Geometry: final body of the model. Coordinates: model frame, mm. Give positions to 0.01 mm unless a question says otherwise; leave off trailing zeros. Order: outer loops, then holes, each group sorted by start corner. A loop starts at its lowest first (then second) coordinate and runs counter-clockwise, first axis right, second up. Notation, with made-up numbers: (61, 65) - (106, 65) arc R15 ccw to (106, 77) - close; hole circle Ø1 at (39.25, -4). An arc over 180 degrees is marked (long way). One line per question, with ' | ' between items. Start each with the question number.
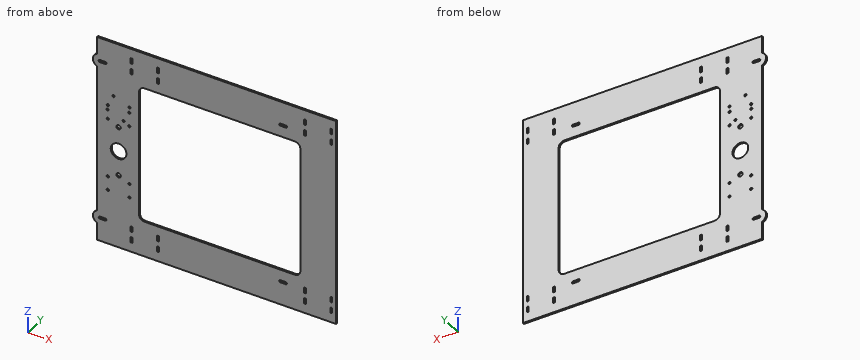
from build123d import *

# Parameters (mm, degrees)
SKETCH1_W           = 434.18
SKETCH1_H           = 380
BOSS_EXTRUDE1_DEPTH = 3
SKETCH2_W           = 250
SKETCH2_H           = 250
CUT_EXTRUDE1_DEPTH  = 4
SKETCH3_W           = 3
SKETCH3_H           = 10
CUT_EXTRUDE2_DEPTH  = 4
SKETCH6_R           = 14.2875
SKETCH6_R_2         = 2
SKETCH6_R_3         = 2.083333333
SKETCH6_R_4         = 4
CUT_EXTRUDE3_DEPTH  = 4
SKETCH7_W           = 83.283399819
SKETCH7_H           = 250
CUT_EXTRUDE4_DEPTH  = 4
FILLET1_R           = 10
CUT_EXTRUDE5_DEPTH  = 4
SKETCH9_R           = 12.5
BOSS_EXTRUDE2_DEPTH = 3


with BuildPart() as part:
    # Sketch1 → Boss-Extrude1 (new body)
    with BuildSketch(Plane(origin=(0, 0, 0), x_dir=(1, 0, 0), z_dir=(0, 1, 0))):
        Rectangle(SKETCH1_W, SKETCH1_H)
    extrude(amount=BOSS_EXTRUDE1_DEPTH)

    # Sketch2 → Cut-Extrude1 (cut, through all)
    with BuildSketch(Plane(origin=(0, 3, 0), x_dir=(1, 0, 0), z_dir=(0, 1, 0))):
        with Locations((27.09, 0)):
            Rectangle(SKETCH2_W, SKETCH2_H)
    extrude(amount=-CUT_EXTRUDE1_DEPTH, mode=Mode.SUBTRACT)

    # Sketch3 → Cut-Extrude2 (cut, through all)
    with BuildSketch(Plane(origin=(0, 3, 0), x_dir=(1, 0, 0), z_dir=(0, 1, 0))):
        with Locations((160.59, -147.5)):
            Rectangle(SKETCH3_W, SKETCH3_H)
        with Locations((160.59, -167.5)):
            Rectangle(SKETCH3_W, SKETCH3_H)
        with Locations((208.59, -147.5)):
            Rectangle(SKETCH3_W, SKETCH3_H)
        with Locations((208.59, -167.5)):
            Rectangle(SKETCH3_W, SKETCH3_H)
        with Locations((-154.41, -147.5)):
            Rectangle(SKETCH3_W, SKETCH3_H)
        with Locations((-154.41, -167.5)):
            Rectangle(SKETCH3_W, SKETCH3_H)
        with Locations((-106.41, -167.5)):
            Rectangle(SKETCH3_W, SKETCH3_H)
        with Locations((-106.41, -147.5)):
            Rectangle(SKETCH3_W, SKETCH3_H)
        with Locations((208.59, 147.5)):
            Rectangle(SKETCH3_W, SKETCH3_H)
        with Locations((208.59, 167.5)):
            Rectangle(SKETCH3_W, SKETCH3_H)
        with Locations((160.59, 167.5)):
            Rectangle(SKETCH3_W, SKETCH3_H)
        with Locations((160.59, 147.5)):
            Rectangle(SKETCH3_W, SKETCH3_H)
        with Locations((-106.41, 147.5)):
            Rectangle(SKETCH3_W, SKETCH3_H)
        with Locations((-106.41, 167.5)):
            Rectangle(SKETCH3_W, SKETCH3_H)
        with Locations((-154.41, 167.5)):
            Rectangle(SKETCH3_W, SKETCH3_H)
        with Locations((-154.41, 147.5)):
            Rectangle(SKETCH3_W, SKETCH3_H)
    extrude(amount=-CUT_EXTRUDE2_DEPTH, mode=Mode.SUBTRACT)

    # Sketch6 → Cut-Extrude3 (cut, through all)
    with BuildSketch(Plane(origin=(0, 3, 0), x_dir=(1, 0, 0), z_dir=(0, 1, 0))):
        with Locations((-177.91, 10)):
            Circle(SKETCH6_R)
        with Locations((-197.793356941, -60.788209542)):
            Circle(SKETCH6_R_2)
        with Locations((-187.137790458, -89.899356941)):
            Circle(SKETCH6_R_2)
        with Locations((-158.026643059, -79.243790458)):
            Circle(SKETCH6_R_2)
        with Locations((-168.682209542, -50.132643059)):
            Circle(SKETCH6_R_2)
        with Locations((-158.345, 64.0505)):
            Circle(SKETCH6_R_3)
        with Locations((-197.475, 64.0505)):
            Circle(SKETCH6_R_3)
        with Locations((-197.475, -44.0505)):
            Circle(SKETCH6_R_3)
        with Locations((-158.345, -44.0505)):
            Circle(SKETCH6_R_3)
        with Locations((-197.475, 89.4505)):
            Circle(SKETCH6_R_3)
        with Locations((-158.345, 89.4505)):
            Circle(SKETCH6_R_3)
        with Locations((-158.345, -69.4505)):
            Circle(SKETCH6_R_3)
        with Locations((-197.475, -69.4505)):
            Circle(SKETCH6_R_3)
        with Locations((-177.91, -35)):
            Circle(SKETCH6_R_4)
        with Locations((-177.91, 55)):
            Circle(SKETCH6_R_4)
    extrude(amount=-CUT_EXTRUDE3_DEPTH, mode=Mode.SUBTRACT)

    # Sketch7 → Cut-Extrude4 (cut, through all)
    with BuildSketch(Plane(origin=(0, 3, 0), x_dir=(1, 0, 0), z_dir=(0, 1, 0))):
        with Locations((-99.169040346, 0)):
            Rectangle(SKETCH7_W, SKETCH7_H)
    extrude(amount=-CUT_EXTRUDE4_DEPTH, mode=Mode.SUBTRACT)

    # Fillet1
    fillet1_edges = [part.edges().sort_by_distance(p)[0] for p in [
        (152.09, 1.5, -125),
        (152.09, 1.5, 125),
        (-140.810740255, 1.5, -125),
        (-140.810740255, 1.5, 125),
    ]]
    fillet(fillet1_edges, radius=FILLET1_R)

    # Sketch8 → Cut-Extrude5 (cut, through all)
    with BuildSketch(Plane(origin=(0, 3, 0), x_dir=(1, 0, 0), z_dir=(0, 1, 0))):
        with BuildLine():
            Line((-212.09, 148.805), (-202.09, 148.805))
            ThreePointArc((-202.09, 148.805), (-200.035, 146.75), (-202.09, 144.695))
            Line((-202.09, 144.695), (-212.09, 144.695))
            ThreePointArc((-212.09, 144.695), (-214.145, 146.75), (-212.09, 148.805))
        make_face()
        with BuildLine():
            Line((-212.09, -144.695), (-202.09, -144.695))
            ThreePointArc((-202.09, -144.695), (-200.035, -146.75), (-202.09, -148.805))
            Line((-202.09, -148.805), (-212.09, -148.805))
            ThreePointArc((-212.09, -148.805), (-214.145, -146.75), (-212.09, -144.695))
        make_face()
        with BuildLine():
            Line((115.91, -144.695), (125.91, -144.695))
            ThreePointArc((125.91, -144.695), (127.965, -146.75), (125.91, -148.805))
            Line((125.91, -148.805), (115.91, -148.805))
            ThreePointArc((115.91, -148.805), (113.855, -146.75), (115.91, -144.695))
        make_face()
        with BuildLine():
            Line((115.91, 148.805), (125.91, 148.805))
            ThreePointArc((125.91, 148.805), (127.965, 146.75), (125.91, 144.695))
            Line((125.91, 144.695), (115.91, 144.695))
            ThreePointArc((115.91, 144.695), (113.855, 146.75), (115.91, 148.805))
        make_face()
    extrude(amount=-CUT_EXTRUDE5_DEPTH, mode=Mode.SUBTRACT)

    # Sketch9 → Boss-Extrude2 (add)
    with BuildSketch(Plane(origin=(0, 3, 0), x_dir=(1, 0, 0), z_dir=(0, 1, 0))):
        with Locations((-212.09, 146.75)):
            Circle(SKETCH9_R)
        with BuildLine():
            ThreePointArc((-212.09, 148.805), (-214.145, 146.75), (-212.09, 144.695))
            Line((-212.09, 144.695), (-202.09, 144.695))
            ThreePointArc((-202.09, 144.695), (-200.035, 146.75), (-202.09, 148.805))
            Line((-202.09, 148.805), (-212.09, 148.805))
        make_face(mode=Mode.SUBTRACT)
        with Locations((-212.09, -146.75)):
            Circle(SKETCH9_R)
        with BuildLine():
            ThreePointArc((-212.09, -144.695), (-214.145, -146.75), (-212.09, -148.805))
            Line((-212.09, -148.805), (-202.09, -148.805))
            ThreePointArc((-202.09, -148.805), (-200.035, -146.75), (-202.09, -144.695))
            Line((-202.09, -144.695), (-212.09, -144.695))
        make_face(mode=Mode.SUBTRACT)
    extrude(amount=-BOSS_EXTRUDE2_DEPTH)


solid = part.part
(1) Cut plane B-B, the plane y = 1. Give the number of separate pieces and of enclosed holes in the cut face, plus the area to 3 significant figures.
(2) Cut plane A-A, the plane z = -10. Return the cut outline in (x, y).
(3) Contact query for a flat-ended pin moving along its axis: P1, Ø0.9, axis at y = 1, z = -168.5, coming from the -X side. Output: stop coordinate, or through.
(4) Material intervals for line 1 along Z through (x, y) = (119.5, 1.95) (3 decimals); line 2 along X through (y, z) = (1.6, -55); line 3 along Z through (x, y) = (65, 1.5), sorted ascending. Write a range as from..to.
Results are:
1) separate pieces: 1 | enclosed holes: 36 | area: 90,500 mm2
2) outline: (-217.09, 0) - (-192.2, 0) - (-192.2, 3) - (-217.09, 3) - close; (-163.62, 0) - (-140.81, 0) - (-140.81, 3) - (-163.62, 3) - close; (152.09, 0) - (217.09, 0) - (217.09, 3) - (152.09, 3) - close
3) P1: x = -217.09
4) line 1: -190..-148.805, -144.695..-125, 125..144.695, 148.805..190 | line 2: -217.09..-181.91, -173.91..-140.81, 152.09..217.09 | line 3: -190..-125, 125..190
